Verification items for the finished model (mm, model axes). Coordinates: 2 decimals unless noted, no trailing zeros. Loops run counter-clockwise (first coordinate to the right, second up) from the corner with the lowest first, then second, coordinate; pieces in that order, holes last. Notation, with made-up numbers: (-35.75, 61) -> (-26.75, 61) arc R24 ccw to (-26.75, 84) -> close; hole circle Ø2 at (22, 72.25). An arc over 180 degrees is marked (long way). Answer as a JSON object with one key per item and string values. Group by question number.
Q1. Cross-section at B-B on z = 31.5. Record the boundary of the cut face in (x, y).
Q2. Scan lines: L1, parallel to X at y = 8.5, z = 22; L2, parallel to Z at x = -45.25, y = 19; L3, parallel to X at y = 21, z = 24.5. Record each from-to range of solid material in increasing order.
Q3. Cross-section at C-C on x = -42. Record the boundary of the cut face in (y, z).
Q4. Cross-section at A-A on y = 10.5. Record the boundary of the cut face in (x, z).
Q5. Gauge pin test, flat end, axial feed: pin 1 Ø1.5 at (x, y) = (-44.5, 27) entering from +Z. Record the tip position at first contact, or that the pin passes through.
```python
from build123d import *

# Parameters (mm, degrees)
BOSS_EXTRUDE1_DEPTH = 48


with BuildPart() as part:
    # Sketch1 → Boss-Extrude1 (new body)
    with BuildSketch(Plane(origin=(0, 0, 0), x_dir=(0.9999530758491465, 0, -0.009687419668383268), z_dir=(0, 1, 0))):
        with BuildLine():
            Line((-41.314383982, -20.77443632), (-46.26820393, -29.461156439))
            ThreePointArc((-46.26820393, -29.461156439), (-42.993051469, -31.13201524), (-39.576799535, -32.491285451))
            Line((-39.576799535, -32.491285451), (-39.2598183, -21.865759848))
            Line((-39.2598183, -21.865759848), (-39.2591075, -21.841933141))
            ThreePointArc((-39.2591075, -21.841933141), (-40.297217765, -21.328346763), (-41.314383982, -20.77443632))
        make_face()
    extrude(amount=BOSS_EXTRUDE1_DEPTH)


solid = part.part
```
Computed values:
{
 "1": {"outline": "(-42.8, 0) -> (-39.23, 0) -> (-39.23, 48) -> (-42.8, 48) -> close"},
 "2": {"L1": "x = -41.57 to -39.52", "L2": "z = 28.6 to 30.31", "L3": "x = -42.97 to -39.09"},
 "3": {"outline": "(0, 22.77) -> (48, 22.77) -> (48, 31.84) -> (0, 31.84) -> close"},
 "4": {"outline": "(-45.98, 29.91) -> (-41.11, 21.17) arc R29.52 cw to (-39.05, 22.22) -> (-39.26, 32.87) arc R39.52 ccw to start"},
 "5": {"pin 1": "stops at z = 31.06"}
}
